Answer from the drawing. Dimensions are ordinates in mm from the lowest x, y and z of the part. A direction names the side the tool comes from. Coordinates: 2 decimals unless noted, no trailing zeros. Write each loop counter-clockwise with the first axis right and the second up, starting at its lowest first coordinate (ties: lowest second). Pieces come first, ordered by that corner, then holes.
(1) The part is cut by section A-A on x = 7. Determine the outline of the cut face in (y, z).
(2) The part is cut by section C-C on z = 5.25. Determine the outline of the cut face in (x, y).
(3) Given P1, Ø2, axis at y = 11.5, z = 4, coming from the -X side; P2, Ø2, axis at y = 10, z = 3.5, coming from the +X side; P3, Ø1.5, axis at y = 10.5, z = 7, coming from the +X side, each flat-ended and moving along its own axis, determine where each tip first touches the part or whether it passes through.
(4) For a pull along Z with two mould halves and no side action, classify the marked faces 3, 4 and 5 as +Z half, -Z half, draft (parallel to the pull), parting line (faces both ways), or undercut.
(5) Straight lines are drawn through the part: line 1 (Z direction, x = 2.5, y = 11.25); line 2 (Y direction, x = 7.5, z = 1.5); line 3 (X direction, y = 5.75, z = 9.25). For each, find the intervals that lie inside material, in ascending order.
(6) The part is cut by section B-B on y = 7.5. Determine the outline of the cut face in (x, z).
(7) The part is cut by section D-D on x = 12.5. Determine the outline of the cut face in (y, z), plus the area to 3 significant figures.
(8) Which of the six approach directions +Z, -Z, +X, -X, +Y, -Y give full straight-line access (tool end or side, diameter ignored) to the marked faces 1 and 2?
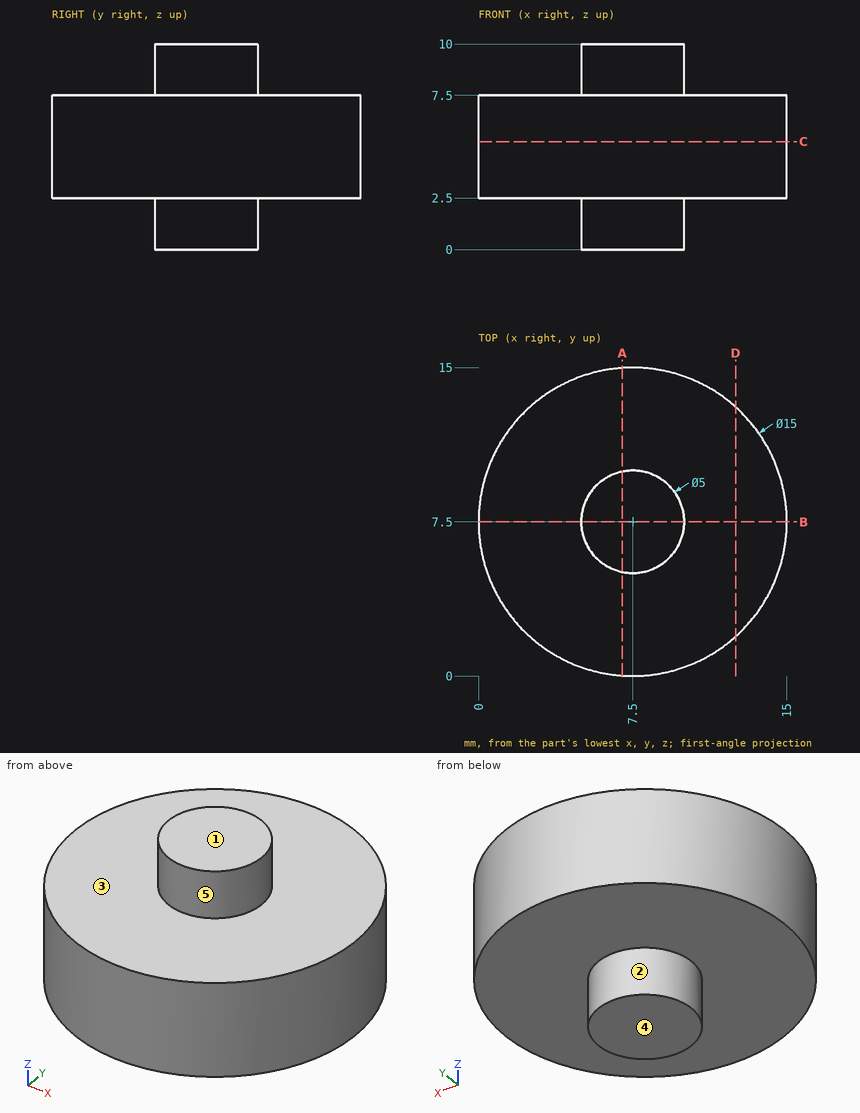
Model answer:
1. outline: (0.02, 2.5) - (5.05, 2.5) - (5.05, 0) - (9.95, 0) - (9.95, 2.5) - (14.98, 2.5) - (14.98, 7.5) - (9.95, 7.5) - (9.95, 10) - (5.05, 10) - (5.05, 7.5) - (0.02, 7.5) - close
2. outline: circle Ø15 at (7.5, 7.5)
3. P1: stops at x = 0.63
3. P2: stops at x = 14.85
3. P3: stops at x = 14.65
4. face 3: +Z half
4. face 4: -Z half
4. face 5: draft
5. line 1: z = 2.5 to 7.5
5. line 2: y = 5 to 10
5. line 3: x = 5.71 to 9.29
6. outline: (0, 2.5) - (5, 2.5) - (5, 0) - (10, 0) - (10, 2.5) - (15, 2.5) - (15, 7.5) - (10, 7.5) - (10, 10) - (5, 10) - (5, 7.5) - (0, 7.5) - close
7. outline: (1.91, 2.5) - (13.09, 2.5) - (13.09, 7.5) - (1.91, 7.5) - close
7. area: 55.9 mm2
8. face 1: +Z, +X, -X, +Y, -Y
8. face 2: -Z
